Input: part model. Units: mm. Frame: model coordinates. Face numbers are marked on the shaded views. A direction names the side the tool comes from. Coordinates: 2 decimals unless noted, no trailing zeros. Loops run counter-clockwise (first coordinate to the right, second up) from the corner with the lowest first, then second, coordinate; pieces in that order, holes last. Notation, with made-up numbers: (68, -22) - (100, -22) arc R24 ccw to (100, 16) - close; hole circle Ø10 at (-1.75, 17.5). An arc over 180 degrees is marked (long way). Use a Markdown table: item, result. Add a question column.
1. Access query for the marked faces 1, 2, 3 and 4. Directions: +Z, -Z, +X, -X, +Y, -Y. A direction counts if a zero-diameter tool reaches every point of the face in a straight line with its end or side. Return the directions, or none.
2. Contact query for flat-ended pins moving along their axis: P1, Ø1.5, axis at x = 9.5, y = 5.5, coming from the -Z side; P2, Ø5, axis at x = 15, z = -6, coming from the +Y side; P3, Ø4, axis at x = 3.5, y = -2, coming from the +Z side; P4, Ø2, axis at y = 4, z = 0.5, coming from the -X side. Output: stop coordinate, or through.
3. Ray query, L1, parallel to Z at x = 7, y = 4.25; L2, parallel to Y at x = 5.75, z = 1.75; L3, parallel to Z at x = -4, y = 6.25. Return the intervals inside material, ascending. Write a range as [from, to].
4. Section query D-D on x = 2. Return the cut outline in (y, z), then the cut area to 3 significant figures.
5. Section query B-B on x = 5.5. Return the cut outline in (y, z).
Autodesk Inventor part; units mm, degrees
ref_plane "YZ Plane" through (0, 0, 0) normal (1, 0, 0) x (0, 1, 0)
ref_plane "XZ Plane" through (0, 0, 0) normal (0, 1, 0) x (-1, 0, 0)
ref_plane "XY Plane" through (0, 0, 0) normal (0, 0, 1) x (1, 0, 0)
sketch "스케치1" plane through (0, 0, 0) normal (0, 0, 1) x (1, 0, 0)
  circle A0 centre (0, 0) radius 3.5
  line L0 (-9, 9) -> (12, 9)
  line L1 (12, 9) -> (12, -9)
  line L2 (12, -9) -> (-9, -9)
  line L3 (-9, -9) -> (-9, 9)
  dimension "d0" = 7
  dimension "d1" = 21
  dimension "d2" = 18
  dimension "d3" = 12
  dimension "d4" = 9
extrude "돌출1" add sketch "스케치1" along normal mid plane 6
extrude "돌출2" add sketch "스케치1" along normal mid plane 15 contours A0
fillet "모깎기1" radius 9 2 edges at (-9, 9, 0) (-9, -9, 0)
chamfer "모따기1" distance 2 angle 45 6 edges at (-6.3641, 6.3641, 3) (5.9998, 9, 3) (5.9998, -9, 3) (-6.3641, 6.3641, -3) (5.9998, -9, -3) (5.9998, 9, -3)
sketch "스케치2" plane through (12, -7, 3) normal (1, 0, 0) x (0, 0, -1)
  circle A0 centre (3, 7) radius 2.5
  dimension "d13" = 5
extrude "돌출3" add sketch "스케치2" along normal blind 6
properties part number "2번부품"
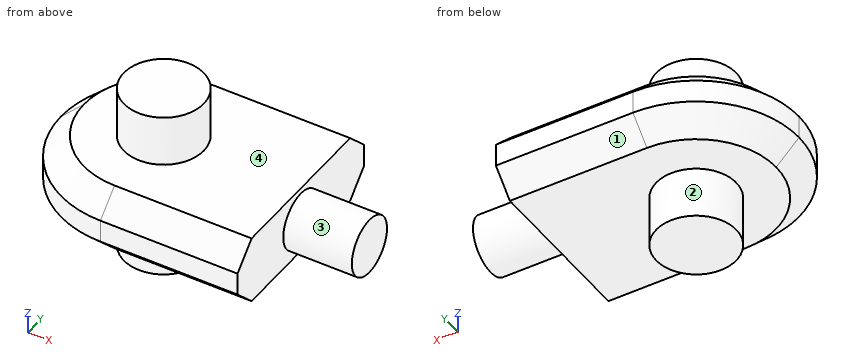
Resolved:
| question | item | result |
|---|---|---|
| 1 | face 1 | -Z, +X, -X, +Y |
| 1 | face 2 | -Z |
| 1 | face 3 | +X |
| 1 | face 4 | +Z |
| 2 | P1 | z = -3 |
| 2 | P2 | through |
| 2 | P3 | z = 7.5 |
| 2 | P4 | x = -8.49 |
| 3 | L1 | [-3, 3] |
| 3 | L2 | [-8.25, 8.25] |
| 3 | L3 | [-2.58, 2.58] |
| 4 | outline | (-9, -1) - (-7, -3) - (-2.87, -3) - (-2.87, -7.5) - (2.87, -7.5) - (2.87, -3) - (7, -3) - (9, -1) - (9, 1) - (7, 3) - (2.87, 3) - (2.87, 7.5) - (-2.87, 7.5) - (-2.87, 3) - (-7, 3) - (-9, 1) - close |
| 4 | area | 152 mm² |
| 5 | outline | (-9, -1) - (-7, -3) - (7, -3) - (9, -1) - (9, 1) - (7, 3) - (-7, 3) - (-9, 1) - close |
